The figure shows three views and two pictorial views of one solid part (mm, origin at its lowest corner). Answer the questions. A direction names the side the tool comes from. Coordinates: 2 decimals unless noted, no trailing zeros. Loops run counter-clockwise (first coordinate to the right, second up) from the corner with the lowest first, then second, coordinate; pieces in that order, holes last. Notation, with made-up numbers: M 44.25,69.25 L 100.25,69.25 A12 ccw 100.25,76.25 Z; hole C -24.75,-20.75 d9. An arc over 180 degrees is marked long. Return JSON: item names as keys, results as strings. Group by question number.
1. Section A-A (z = 166) is taken. Write down the section's boundary in (x, y).
2. Section B-B (x = 34.5) is taken. Write down the section's boundary in (y, z).
3. Straight lines are drawn through the part: L1, parallel to X at y = 262, z = 153.5; L2, parallel to Y at x = 73.5, z = 23.5. For each, find the intervals that lie inside material, in ascending order. Write a range as from..to.
4. Given P1, Ø12, axis at x = 69, z = 87.5, coming from the -Y side; P2, Ø12.5, axis at y = 279.5, z = 89.5, coming from the +X side; P3, Ø2, axis at x = 229.5, z = 180, coming from the -Y side; P4, Ø3, axis at x = 143.5, y = 37, coming from the -Z side, each flat-ended and moving along its own axis, determine where each tip first touches the part or whether it passes through.
5. Which of the six approach directions +Z, -Z, +X, -X, +Y, -Y give full straight-line access (tool end or side, diameter ignored) to the marked faces 1, 2 and 3?
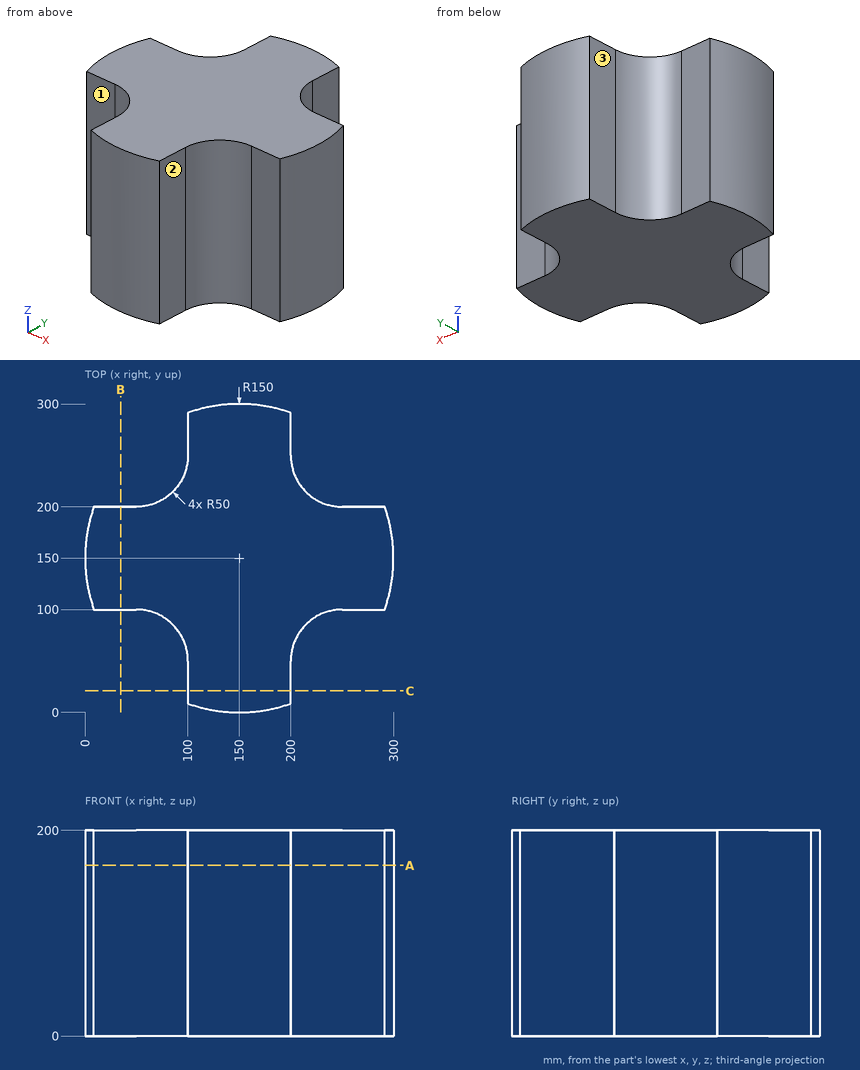
Worked out:
{
 "1": {"outline": "M 8.58,100 L 50,100 A50 cw 100,50 L 100,8.58 A150 ccw 200,8.58 L 200,50 A50 cw 250,100 L 291.42,100 A150 ccw 291.42,200 L 250,200 A50 cw 200,250 L 200,291.42 A150 ccw 100,291.42 L 100,250 A50 cw 50,200 L 8.58,200 A150 ccw Z"},
 "2": {"outline": "M 100,0 L 200,0 L 200,200 L 100,200 Z"},
 "3": {"L1": "100..200", "L2": "94.13..205.87"},
 "4": {"P1": "y = 93.3", "P2": "x = 200", "P3": "y = 95.14", "P4": "z = 0"},
 "5": {"face 1": "+Z, -Z, -X, -Y", "face 2": "+Z, -Z, +X, -Y", "face 3": "+Z, -Z, -X, +Y"}
}
